```python
from build123d import *

# Parameters (mm, degrees)
F0_R     = 49.325
F1_DEPTH = 35
F2_R     = 50.949496
F2_R_2   = 43.141888
F3_DEPTH = 25
F4_R     = 28.5
F5_DEPTH = 35


with BuildPart() as f1:
    # F0 (on Front) → F1 (new body)
    with BuildSketch(Plane.XZ):
        Circle(F0_R)
    extrude(amount=F1_DEPTH)

    # F2 (on face) → F3 (cut)
    with BuildSketch(Plane.XZ.offset(35)):
        Circle(F2_R)
        Circle(F2_R_2, mode=Mode.SUBTRACT)
    extrude(amount=-F3_DEPTH, mode=Mode.SUBTRACT)

    # F4 (on face) → F5 (join)
    with BuildSketch(Plane.XZ.offset(35)):
        Circle(F4_R)
    extrude(amount=F5_DEPTH)


solid = f1.part
```
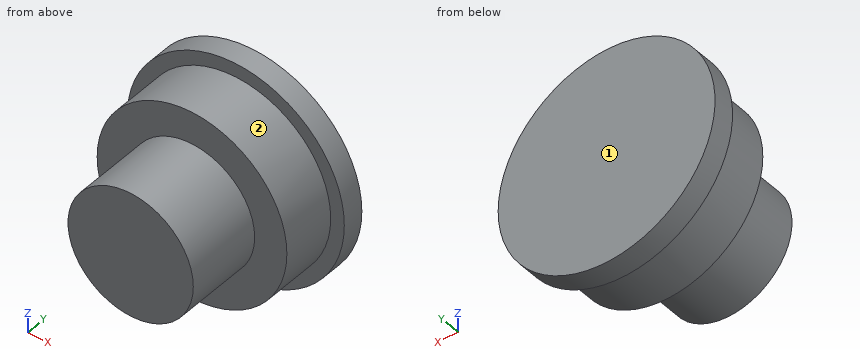
Build history of the part. All positions in model axes, mm. Face numbers are marked on the shaded views. A direction names the side the tool comes from. Give positions to 0.01 mm unless a question says otherwise; leave off trailing zeros. Loops run counter-clockwise (first coordinate to the right, second up) from the corner with the lowest first, then second, coordinate; pieces in that order, holes last.
1) 3-axis set-ups, long thin cutter, end or side, ignore diameter. For the marked faces 1 and 2: which of +Z, -Z, +X, -X, +Y, -Y reach the whole face in a straight line?
Values follow:
face 1: +Z, -Z, +X, -X, +Y
face 2: -Y
2) Probe line 1 along X through (y, z) = (-64.5, -1); line 2 along Y through (x, z) = (-33.5, -8); line 3 along Z through (x, y) = (20.5, -33.5). List the from-to ranges inside material, lowest first.
Values follow:
line 1: x = -28.48 to 28.48
line 2: y = -35 to 0
line 3: z = -37.96 to 37.96
3) Drop flat-ended pins along their axis: P1, Ø1.5, axis at x = 13, z = -34, coming from the -Y side; P2, Ø4, axis at x = 39, y = -22.5, coming from the -Z side; P3, Ø10, axis at y = -53, z = 7, coming from the +X side; P4, Ø5, axis at y = -39.5, z = 32, coming from the -X side. Give the stop position or say it passes through.
Values follow:
P1: stops at y = -35
P2: stops at z = -22.19
P3: stops at x = 28.43
P4: passes through
4) Band-saw the part on D-D on x = 32. List the corners of the cut face in (y, z), then the cut area to 3 significant figures.
Values follow:
outline: (-35, -28.93) - (-10, -28.93) - (-10, -37.54) - (0, -37.54) - (0, 37.54) - (-10, 37.54) - (-10, 28.93) - (-35, 28.93) - close
area: 2,200 mm2
5) Band-saw the part on A-A on x = 0. List the corners of the cut face in (y, z) (3 decimals).
Values follow:
outline: (-70, -28.5) - (-35, -28.5) - (-35, -43.142) - (-10, -43.142) - (-10, -49.325) - (0, -49.325) - (0, 49.325) - (-10, 49.325) - (-10, 43.142) - (-35, 43.142) - (-35, 28.5) - (-70, 28.5) - close
6) Band-saw the part on B-B on z = 0. List the corners of the cut face in (x, y) (3 decimals).
Values follow:
outline: (-49.325, -10) - (-43.142, -10) - (-43.142, -35) - (-28.5, -35) - (-28.5, -70) - (28.5, -70) - (28.5, -35) - (43.142, -35) - (43.142, -10) - (49.325, -10) - (49.325, 0) - (-49.325, 0) - close
7) Band-saw the part on C-C on y = -8.5. List the corners of the cut face in (x, z) (3 decimals), then the cut area to 3 significant figures.
Values follow:
outline: circle Ø98.65 at (0, 0)
area: 7,640 mm2
